from build123d import *

# Parameters (mm, degrees)
SKETCH_1_R          = 1.65
EXTRUDE_1_DEPTH     = 3
SKETCH_3_R          = 1.65
CUT_EXTRUDE_2_DEPTH = 109.673823895
SKETCH_4_R          = 1.65
CUT_EXTRUDE_3_DEPTH = 109.673823895
CUT_EXTRUDE_4_DEPTH = 109.673823895


with BuildPart() as part:
    # Эскиз1 → Бобышка-Вытянуть1 (new body)
    with BuildSketch(Plane.XY):
        with BuildLine():
            Line((-34, 101), (34, 101))
            ThreePointArc((34, 101), (38.242640687, 99.242640687), (40, 95))
            Line((40, 95), (40, -95))
            ThreePointArc((40, -95), (38.242640687, -99.242640687), (34, -101))
            Line((34, -101), (-34, -101))
            ThreePointArc((-34, -101), (-38.242640687, -99.242640687), (-40, -95))
            Line((-40, -95), (-40, 95))
            ThreePointArc((-40, 95), (-38.242640687, 99.242640687), (-34, 101))
        make_face()
        with Locations((-35, 91)):
            Circle(SKETCH_1_R, mode=Mode.SUBTRACT)
        with Locations((-35, 35)):
            Circle(SKETCH_1_R, mode=Mode.SUBTRACT)
        with Locations(Location((35, 35, 0), (0, 0, 180))):
            Circle(SKETCH_1_R, mode=Mode.SUBTRACT)
        with Locations(Location((35, 91, 0), (0, 0, 180))):
            Circle(SKETCH_1_R, mode=Mode.SUBTRACT)
        with Locations((35, -91)):
            Circle(SKETCH_1_R, mode=Mode.SUBTRACT)
        with Locations(Location((-35, -91, 0), (0, 0, 180))):
            Circle(SKETCH_1_R, mode=Mode.SUBTRACT)
        with Locations(Location((-35, -35, 0), (0, 0, 180))):
            Circle(SKETCH_1_R, mode=Mode.SUBTRACT)
        with Locations((35, -35)):
            Circle(SKETCH_1_R, mode=Mode.SUBTRACT)
    extrude(amount=EXTRUDE_1_DEPTH)

    # Эскиз3 → Вырез-Вытянуть2 (cut, through all)
    with BuildSketch(Plane.XY.offset(3)):
        with Locations((-24.5, -93.5)):
            Circle(SKETCH_3_R)
        with Locations((-24.5, -35.5)):
            Circle(SKETCH_3_R)
        with Locations((-15.25, 1.25)):
            Circle(SKETCH_3_R)
        with Locations((-15.25, 31.75)):
            Circle(SKETCH_3_R)
        with Locations((-26, 44)):
            Circle(SKETCH_3_R)
        with Locations((-26, 96)):
            Circle(SKETCH_3_R)
        with Locations(Location((24.5, -93.5, 0), (0, 0, 180))):
            Circle(SKETCH_3_R)
        with Locations(Location((24.5, -35.5, 0), (0, 0, 180))):
            Circle(SKETCH_3_R)
        with Locations(Location((15.25, 1.25, 0), (0, 0, 180))):
            Circle(SKETCH_3_R)
        with Locations(Location((15.25, 31.75, 0), (0, 0, 180))):
            Circle(SKETCH_3_R)
        with Locations(Location((26, 44, 0), (0, 0, 180))):
            Circle(SKETCH_3_R)
        with Locations(Location((26, 96, 0), (0, 0, 180))):
            Circle(SKETCH_3_R)
    extrude(amount=-CUT_EXTRUDE_2_DEPTH, mode=Mode.SUBTRACT)

    # Эскиз4 → Вырез-Вытянуть3 (cut, through all)
    with BuildSketch(Plane.XY.offset(3)):
        with Locations((-35, 76.19)):
            Circle(SKETCH_4_R)
        with Locations(Location((35, 76.19, 0), (0, 0, 180))):
            Circle(SKETCH_4_R)
        with Locations((35, -76.19)):
            Circle(SKETCH_4_R)
        with Locations(Location((-35, -76.19, 0), (0, 0, 180))):
            Circle(SKETCH_4_R)
    extrude(amount=-CUT_EXTRUDE_3_DEPTH, mode=Mode.SUBTRACT)

    # Эскиз5 → Вырез-Вытянуть4 (cut, through all)
    with BuildSketch(Plane.XY.offset(3)):
        with BuildLine():
            Line((-33.5, 14.365), (-33.5, -14.365))
            ThreePointArc((-33.5, -14.365), (-35, -15.865), (-36.5, -14.365))
            Line((-36.5, -14.365), (-36.5, 14.365))
            ThreePointArc((-36.5, 14.365), (-35, 15.865), (-33.5, 14.365))
        make_face()
        with BuildLine():
            Line((-25.49, 18.895), (-25.49, -18.895))
            ThreePointArc((-25.49, -18.895), (-26.99, -20.395), (-28.49, -18.895))
            Line((-28.49, -18.895), (-28.49, 18.895))
            ThreePointArc((-28.49, 18.895), (-26.99, 20.395), (-25.49, 18.895))
        make_face()
        with BuildLine():
            Line((-16.5, -41.32), (-16.5, -86.32))
            ThreePointArc((-16.5, -86.32), (-18, -87.82), (-19.5, -86.32))
            Line((-19.5, -86.32), (-19.5, -41.32))
            ThreePointArc((-19.5, -41.32), (-18, -39.82), (-16.5, -41.32))
        make_face()
        with BuildLine():
            Line((-8.5, -23.74), (-8.5, -86.32))
            ThreePointArc((-8.5, -86.32), (-10, -87.82), (-11.5, -86.32))
            Line((-11.5, -86.32), (-11.5, -23.74))
            ThreePointArc((-11.5, -23.74), (-10, -22.24), (-8.5, -23.74))
        make_face()
        with BuildLine():
            Line((1.5, -15.03), (1.5, -95.03))
            ThreePointArc((1.5, -95.03), (0, -96.53), (-1.5, -95.03))
            Line((-1.5, -95.03), (-1.5, -15.03))
            ThreePointArc((-1.5, -15.03), (0, -13.53), (1.5, -15.03))
        make_face()
        with BuildLine():
            Line((8.5, -23.74), (8.5, -86.32))
            ThreePointArc((8.5, -86.32), (10, -87.82), (11.5, -86.32))
            Line((11.5, -86.32), (11.5, -23.74))
            ThreePointArc((11.5, -23.74), (10, -22.24), (8.5, -23.74))
        make_face()
        with BuildLine():
            Line((16.5, -41.32), (16.5, -86.32))
            ThreePointArc((16.5, -86.32), (18, -87.82), (19.5, -86.32))
            Line((19.5, -86.32), (19.5, -41.32))
            ThreePointArc((19.5, -41.32), (18, -39.82), (16.5, -41.32))
        make_face()
        with BuildLine():
            Line((25.49, 18.895), (25.49, -18.895))
            ThreePointArc((25.49, -18.895), (26.99, -20.395), (28.49, -18.895))
            Line((28.49, -18.895), (28.49, 18.895))
            ThreePointArc((28.49, 18.895), (26.99, 20.395), (25.49, 18.895))
        make_face()
        with BuildLine():
            Line((33.5, 14.365), (33.5, -14.365))
            ThreePointArc((33.5, -14.365), (35, -15.865), (36.5, -14.365))
            Line((36.5, -14.365), (36.5, 14.365))
            ThreePointArc((36.5, 14.365), (35, 15.865), (33.5, 14.365))
        make_face()
        with BuildLine():
            Line((-16.5, 41.32), (-16.5, 86.32))
            ThreePointArc((-16.5, 86.32), (-18, 87.82), (-19.5, 86.32))
            Line((-19.5, 86.32), (-19.5, 41.32))
            ThreePointArc((-19.5, 41.32), (-18, 39.82), (-16.5, 41.32))
        make_face()
        with BuildLine():
            Line((-8.5, 23.74), (-8.5, 86.32))
            ThreePointArc((-8.5, 86.32), (-10, 87.82), (-11.5, 86.32))
            Line((-11.5, 86.32), (-11.5, 23.74))
            ThreePointArc((-11.5, 23.74), (-10, 22.24), (-8.5, 23.74))
        make_face()
        with BuildLine():
            Line((8.5, 23.74), (8.5, 86.32))
            ThreePointArc((8.5, 86.32), (10, 87.82), (11.5, 86.32))
            Line((11.5, 86.32), (11.5, 23.74))
            ThreePointArc((11.5, 23.74), (10, 22.24), (8.5, 23.74))
        make_face()
        with BuildLine():
            Line((16.5, 41.32), (16.5, 86.32))
            ThreePointArc((16.5, 86.32), (18, 87.82), (19.5, 86.32))
            Line((19.5, 86.32), (19.5, 41.32))
            ThreePointArc((19.5, 41.32), (18, 39.82), (16.5, 41.32))
        make_face()
        with BuildLine():
            Line((1.5, 15.03), (1.5, 95.03))
            ThreePointArc((1.5, 95.03), (0, 96.53), (-1.5, 95.03))
            Line((-1.5, 95.03), (-1.5, 15.03))
            ThreePointArc((-1.5, 15.03), (0, 13.53), (1.5, 15.03))
        make_face()
    extrude(amount=-CUT_EXTRUDE_4_DEPTH, mode=Mode.SUBTRACT)


solid = part.part
Input: part model. Units: mm. Frame: model coordinates. Round coordinates to 2 decimals unless told otherwise and drop trailing zeros. Order: outer loops, then holes, each group sorted by start corner. A loop starts at its lowest first (then second) coordinate and runs counter-clockwise, first axis right, second up. Notation, with made-up numbers: (-18, -24.5) - (22, -24.5) arc R20 ccw to (22, -9.5) - close; hole circle Ø4 at (59, 53). An arc over 180 degrees is marked (long way). Answer as a JSON object with one key per item and string values. Group by question number.
(1) Draft query along Z for faces 1 (the face through (1, 1, 0)), 2 (the face through (1, 1, 3)), 3 (the face through (-34.6, -89.4, 1.5)). Return one class per face: released by +Z, released by -Z, zero draft, split by the parting line, or undercut.
(2) Cut plane A-A (y = 84). Return loops of the section in (x, z), then the cut area to 3 significant figures.
(3) Material intervals for probe 1 along X at (y, z) = (-51, 0.2); probe 2 along X at (y, z) = (-12.5, 1.3); probe 3 along X at (y, z) = (-93.5, 1.95), sorted ascending. Write a range as from..to.
(4) Cut plane B-B (z = 0.5). Count the separate pieces of the cut face and the enclosed holes in it, then the cut area to 3 significant figures.
Here are the results:
{
 "1": {"face 1": "released by -Z", "face 2": "released by +Z", "face 3": "zero draft"},
 "2": {"outline": "(-40, 0) - (-19.5, 0) - (-19.5, 3) - (-40, 3) - close; (-16.5, 0) - (-11.5, 0) - (-11.5, 3) - (-16.5, 3) - close; (-8.5, 0) - (-1.5, 0) - (-1.5, 3) - (-8.5, 3) - close; (1.5, 0) - (8.5, 0) - (8.5, 3) - (1.5, 3) - close; (11.5, 0) - (16.5, 0) - (16.5, 3) - (11.5, 3) - close; (19.5, 0) - (40, 0) - (40, 3) - (19.5, 3) - close", "area": "195 mm^2"},
 "3": {"probe 1": "x = -40..-19.5, -16.5..-11.5, -8.5..-1.5, 1.5..8.5, 11.5..16.5, 19.5..40", "probe 2": "x = -40..-36.5, -33.5..-28.49, -25.49..25.49, 28.49..33.5, 36.5..40", "probe 3": "x = -40..-26.15, -22.85..-1.5, 1.5..22.85, 26.15..40"},
 "4": {"separate pieces": "1", "enclosed holes": "38", "area": "13,700 mm^2"}
}
